from build123d import *

# Parameters (mm, degrees)
F0_R     = 15.875
F0_R_2   = 9.525
F1_DEPTH = 6.35
F2_DEPTH = 68.58
F3_SIZE2 = 1.27
F3_SIZE  = 1.27
F5_R     = 2.3876
F6_DEPTH = 25.401


with BuildPart() as f1:
    # F0 (on Right) → F1 (new body)
    with BuildSketch(Plane.YZ):
        Circle(F0_R)
        Circle(F0_R_2, mode=Mode.SUBTRACT)
    extrude(amount=F1_DEPTH)

    # F0 (on Right) → F2 (join)
    with BuildSketch(Plane.YZ):
        Circle(F0_R_2)
    extrude(amount=F2_DEPTH)

    # F3
    f3_edges = [f1.edges().sort_by_distance(p)[0] for p in [
        (68.58, -9.525, 0),
    ]]
    chamfer(f3_edges, length=F3_SIZE, length2=F3_SIZE2)

    # F5 (on offset) → F6 (cut, through all)
    with BuildSketch(Plane.XY.offset(9.525)):
        with Locations((62.23, 0)):
            Circle(F5_R)
    extrude(amount=-F6_DEPTH, mode=Mode.SUBTRACT)


solid = f1.part
Model file for the job. Use its own axes, mm. A direction names the side the tool comes from. Give positions to 0.01 mm unless a question says otherwise; leave off trailing zeros. Loops run counter-clockwise (first coordinate to the right, second up) from the corner with the lowest first, then second, coordinate; pieces in that order, holes last. Notation, with made-up numbers: (43, -13.5) -> (100, -13.5) arc R23 cw to (100, 12.5) -> close; hole circle Ø5 at (45, 67.25). An arc over 180 degrees is marked (long way). Use a Markdown table: item, result. Add a question column.
(1) Wall check: line 1 along X through (y, z) = (0, -2.75); line 2 along Y through (x, z) = (62.23, 3); line 3 along X through (y, z) = (-11.5, -10.5). Give the ranges that are in metal, low to high.
(2) Tool access for faces 4 (the flat face through (0, 0, 0)), 5 (the flat face through (6.35, 7, -7)): list every direction of +Z, -Z, +X, -X, +Y, -Y with a clear straight run to the whole face (end or side of a thin tool).
(3) Slice it at D-D on x = 11.5. List the corners of the cut face in (y, z) (3 decimals).
(4) Slice it at B-B on z = 0. List the corners of the cut face in (x, y) (3 decimals), and give its area (3 significant figures).
(5) Slice it at A-A on y = 0. List the corners of the cut face in (x, z) (3 decimals).
(6) Mould opens along X. For faces 1 (the cylindrical face through (59.845, 0.105, 0.13)), 2 (the cylindrical face through (3.131, -3.441, -15.497)), 3 (the flat face through (68.58, 0, 0)) say: +X half, -X half, draft (parallel to the pull), parting line (faces both ways), or undercut.
(7) Drop flat-ended pins along their axis: pin 1 Ø4 at (x, z) = (55, 7.5) entering from +Y; pin 2 Ø1 at (x, y) = (34.5, 1) entering from -Z; pin 3 Ø2 at (x, z) = (53.5, 9.5) entering from -Y; pin 4 Ø4.5 at (x, y) = (62.23, 0) entering from -Z. Give the stop position or say it passes through.
(8) Slice it at C-C on x = 62.23. List the corners of the cut face in (y, z) (3 decimals).
Filled sheet:
| question | item | result |
|---|---|---|
| 1 | line 1 | 0 to 59.84, 64.62 to 68.58 |
| 1 | line 2 | -9.04 to -2.39, 2.39 to 9.04 |
| 1 | line 3 | 0 to 6.35 |
| 2 | face 4 | +Z, -Z, -X, +Y, -Y |
| 2 | face 5 | +X |
| 3 | outline | circle Ø19.05 at (0, 0) |
| 4 | outline | (0, -15.875) -> (6.35, -15.875) -> (6.35, -9.525) -> (67.31, -9.525) -> (68.58, -8.255) -> (68.58, 8.255) -> (67.31, 9.525) -> (6.35, 9.525) -> (6.35, 15.875) -> (0, 15.875) -> close; hole circle Ø4.775 at (62.23, 0) |
| 4 | area | 1,370 mm2 |
| 5 | outline | (0, -15.875) -> (6.35, -15.875) -> (6.35, -9.525) -> (59.842, -9.525) -> (59.842, 9.525) -> (6.35, 9.525) -> (6.35, 15.875) -> (0, 15.875) -> close; (64.618, -9.525) -> (67.31, -9.525) -> (68.58, -8.255) -> (68.58, 8.255) -> (67.31, 9.525) -> (64.618, 9.525) -> close |
| 6 | face 1 | undercut |
| 6 | face 2 | draft |
| 6 | face 3 | +X half |
| 7 | pin 1 | y = 7.78 |
| 7 | pin 2 | z = -9.51 |
| 7 | pin 3 | y = -4.3 |
| 7 | pin 4 | through |
| 8 | outline | (-2.388, -9.221) -> (-2.388, 9.221) arc R9.525 ccw to start; (2.388, -9.221) arc R9.525 ccw to (2.388, 9.221) -> close |
